Autodesk Inventor part; units mm, degrees
ref_plane "YZ Plane" through (0, 0, 0) normal (1, 0, 0) x (0, 1, 0)
ref_plane "XZ Plane" through (0, 0, 0) normal (0, 1, 0) x (-1, 0, 0)
ref_plane "XY Plane" through (0, 0, 0) normal (0, 0, 1) x (1, 0, 0)
sketch "Sketch1" plane through (0, 0, 0) normal (0, 0, 1) x (1, 0, 0)
  line L0 (0, 0) -> (0, 33)
  line L1 (0, 33) -> (3, 33)
  line L2 (3, 33) -> (3, 30)
  line L3 (3, 30) -> (1.5, 30)
  line L4 (1.5, 30) -> (1.5, 0)
  line L5 (1.5, 0) -> (0, 0)
  dimension "d0" = 30
  dimension "d1" = 1.5
  dimension "d2" = 3
  dimension "d3" = 3
revolve "Revolution1" add sketch "Sketch1" angle 360 about axis through (0, 0, 0) along (0, 1, 0)
sketch "Sketch2" plane through (0, 33, 0) normal (0, 1, 0) x (1, 0, 0)
  line L0 (0.7217, 1.25) -> (1.4434, 0)
  line L1 (1.4434, 0) -> (0.7217, -1.25)
  line L2 (0.7217, -1.25) -> (-0.7217, -1.25)
  line L3 (-0.7217, -1.25) -> (-1.4434, 0)
  line L4 (-1.4434, 0) -> (-0.7217, 1.25)
  line L5 (-0.7217, 1.25) -> (0.7217, 1.25)
  point P0 (0, 0)
  point P1 (0, 0)
  dimension "d5" = 2.5
extrude "Extrusion1" cut sketch "Sketch2" against normal blind 3
chamfer "Chamfer1" distance 0.5 angle 45 2 edges at (-3, 30, 0) (-1.5, 0, 0)
properties part number "M3x30 SHCS"
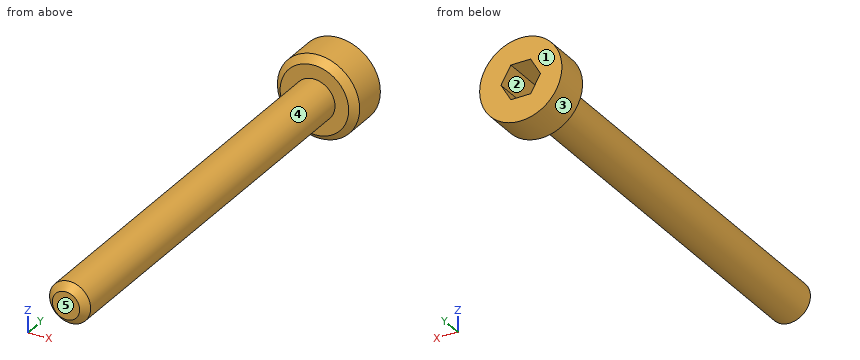
Work out the finished part from the listing and answer in its coordinate system (mm). Face numbers are marked on the shaded views. A direction names the side the tool comes from. Round coordinates to 2 decimals unless told otherwise and drop trailing zeros. Write each loop counter-clockwise with the first axis right and the second up, starting at its lowest first coordinate (ties: lowest second). Pieces come first, ordered by that corner, then holes. Notation, with made-up numbers: (55.5, -26.75) - (100.5, -26.75) arc R16 cw to (100.5, 0.25) - close; hole circle Ø10 at (-9.5, -8.75). An arc over 180 degrees is marked (long way). Return JSON: item names as keys, results as strings. Group by question number.
Q1. The mould has two halves that part along Z. Classify the marked faces 1, 2 and 3: released by +Z, released by -Z, zero draft, split by the parting line, or undercut.
Q2. For the marked faces 4 and 5, determine the directions among +Z, -Z, +X, -X, +Y, -Y from which every point of the face is accessible in a straight line to the end or side of a thin tool.
Q3. Find the intervals of material crossed by L1, parallel to Y at x = -0.35, z = 0.75; L2, parallel to Z at x = 0.1, y = 17; L3, parallel to X at y = 26, z = 0.15, in increasing order.
Q4. The part is cut by section B-B on y = 5. Write down the section's boundary in (x, z).
Q5. The part is cut by section A-A on x = 0. Write down the section's boundary in (y, z), then the cut area to 3 significant figures.
Q6. Each of these flat-tipped pins is pushed along its axis until it touches: pin 1 Ø1.3 at (x, z) = (0.5, 0) entering from +Y; pin 2 Ø1.5 at (x, y) = (-0.5, 26) entering from -Z; pin 3 Ø1.5 at (y, z) = (8.5, 1.5) entering from +X. Where does it stop, or does it pass through?
Solved:
{
 "1": {"face 1": "zero draft", "face 2": "undercut", "face 3": "split by the parting line"},
 "2": {"face 4": "-Y", "face 5": "+Z, -Z, +X, -X, -Y"},
 "3": {"L1": "0 to 30", "L2": "-1.5 to 1.5", "L3": "-1.49 to 1.49"},
 "4": {"outline": "circle Ø3 at (0, 0)"},
 "5": {"outline": "(0, -1) - (0.5, -1.5) - (30, -1.5) - (30, -2.5) - (30.5, -3) - (33, -3) - (33, -1.25) - (30, -1.25) - (30, 1.25) - (33, 1.25) - (33, 3) - (30.5, 3) - (30, 2.5) - (30, 1.5) - (0.5, 1.5) - (0, 1) - close", "area": "100 mm²"},
 "6": {"pin 1": "y = 30", "pin 2": "z = -1.5", "pin 3": "x = 1.3"}
}
